```python
from build123d import *

# Parameters (mm, degrees)
SKETCH2_W           = 190
SKETCH2_H           = 22
BOSS_EXTRUDE1_DEPTH = 32
SKETCH3_R           = 0.75
SKETCH3_R_2         = 6
SKETCH3_R_3         = 3
SKETCH3_W           = 25
SKETCH3_H           = 4
CUT_EXTRUDE1_DEPTH  = 24
SKETCH4_W           = 25
SKETCH4_H           = 4
CUT_EXTRUDE2_DEPTH  = 9
SKETCH5_R           = 3
SKETCH5_R_2         = 2
SKETCH5_R_3         = 6.5
CUT_EXTRUDE3_DEPTH  = 24


with BuildPart() as part:
    # Sketch2 → Boss-Extrude1 (new body)
    with BuildSketch(Plane(origin=(0, 0, 0), x_dir=(1, 0, 0), z_dir=(0, 1, 0))):
        Rectangle(SKETCH2_W, SKETCH2_H)
    extrude(amount=BOSS_EXTRUDE1_DEPTH)

    # Sketch3 → Cut-Extrude1 (cut)
    with BuildSketch(Plane(origin=(0, 32, 0), x_dir=(1, 0, 0), z_dir=(0, 1, 0))):
        with Locations((-87, 0)):
            Circle(SKETCH3_R)
        with Locations((-63, 0)):
            Circle(SKETCH3_R_2)
        with Locations((-37, 5)):
            Circle(SKETCH3_R_3)
        with Locations((-43, 0)):
            Circle(SKETCH3_R)
        with Locations((11, 0)):
            Circle(SKETCH3_R_2)
        with Locations((37, 5)):
            Circle(SKETCH3_R_3)
        with Locations((79.5, 9)):
            Rectangle(SKETCH3_W, SKETCH3_H)
    extrude(amount=-CUT_EXTRUDE1_DEPTH, mode=Mode.SUBTRACT)

    # Sketch4 → Cut-Extrude2 (cut, through all)
    with BuildSketch(Plane(origin=(0, 8, 0), x_dir=(1, 0, 0), z_dir=(0, 1, 0))):
        with Locations((79.5, 9)):
            Rectangle(SKETCH4_W, SKETCH4_H)
    extrude(amount=-CUT_EXTRUDE2_DEPTH, mode=Mode.SUBTRACT)

    # Sketch5 → Cut-Extrude3 (cut)
    with BuildSketch(Plane.XY.offset(11)):
        with Locations((-87, 22)):
            Circle(SKETCH5_R)
        with Locations((-63, 20)):
            Circle(SKETCH5_R_2)
        with Locations((11, 20)):
            Circle(SKETCH5_R_2)
        with Locations((79.5, 20)):
            Circle(SKETCH5_R_3)
    extrude(amount=-CUT_EXTRUDE3_DEPTH, mode=Mode.SUBTRACT)


solid = part.part
```
Geometry check sheet. Reference: the model listing, model coordinates, mm. A direction names the side the tool comes from. Round coordinates to 2 decimals unless told otherwise and drop trailing zeros. Loops run counter-clockwise (first coordinate to the right, second up) from the corner with the lowest first, then second, coordinate; pieces in that order, holes last. Notation, with made-up numbers: (61, 57.5) -> (97, 57.5) arc R27 ccw to (97, 78.5) -> close; hole circle Ø7 at (54.25, 76.25). An arc over 180 degrees is marked (long way). Use a Markdown table: item, result.
(1) Sectioned sample at B-B (y = 3.5). Enter the section's corners in (x, z).
Calculated:
| item | result |
|---|---|
| outline | (-95, -11) -> (67, -11) -> (67, -7) -> (92, -7) -> (92, -11) -> (95, -11) -> (95, 11) -> (-95, 11) -> close |
(2) Mould release check, pull along X, two halves, no side actions. Record for faces 4 (the flat face through (95, 16, 0)), 5 (the flat face through (-95, 16, 0)), 6 (the flat face through (-1, 32, 0)), 7 (the cylindrical face through (11, 18, 8)): released by +X, released by -X, zero draft, split by the parting line, or undercut.
Calculated:
| item | result |
|---|---|
| face 4 | released by +X |
| face 5 | released by -X |
| face 6 | zero draft |
| face 7 | undercut |
(3) Set-up check for faces 1 (the flat face through (-37, 8, -5)), 2 (the cylindrical face through (-62.077, 18.226, 8.366)), 3 (the flat face through (92, 16, -9)): record each of +Z, -Z, +X, -X, +Y, -Y from which the full face is reachable in a straight line by a thin tool's end or side.
Calculated:
| item | result |
|---|---|
| face 1 | +Y |
| face 2 | +Z, -Z |
| face 3 | -Z, +Y, -Y |
(4) Sectioned sample at C-C (x = 37). Enter the section's corners in (y, z).
Calculated:
| item | result |
|---|---|
| outline | (0, -11) -> (32, -11) -> (32, -8) -> (8, -8) -> (8, -2) -> (32, -2) -> (32, 11) -> (0, 11) -> close |
(5) Sectioned sample at A-A (x = 11). Enter the section's corners in (y, z), then the cut area to 3 significant figures.
Calculated:
| item | result |
|---|---|
| outline | (0, -11) -> (18, -11) -> (18, -6) -> (8, -6) -> (8, 6) -> (18, 6) -> (18, 11) -> (0, 11) -> close; (22, -11) -> (32, -11) -> (32, -6) -> (22, -6) -> close; (22, 6) -> (32, 6) -> (32, 11) -> (22, 11) -> close |
| area | 376 mm² |
(6) Go/stop test with flat-tipped pins: P1, Ø1.2, axis at x = -43, z = 0, coming from the -Y side; P2, Ø9.5, axis at x = -63.5, z = 1, coming from the +Y side. Record where each tip stops, or that it passes through.
Calculated:
| item | result |
|---|---|
| P1 | y = 0 |
| P2 | y = 8 |
(7) Scan lines: probe 1 along X at (y, z) = (12, 0); probe 2 along X at (y, z) = (16, -5); probe 3 along Z at (x, y) = (37, 25.75). Record each from-to range of solid material in increasing order.
Calculated:
| item | result |
|---|---|
| probe 1 | -95 to -87.75, -86.25 to -69, -57 to -43.75, -42.25 to 5, 17 to 95 |
| probe 2 | -95 to -66.32, -59.68 to -40, -34 to 7.68, 14.32 to 34, 40 to 74.38, 84.62 to 95 |
| probe 3 | -11 to -8, -2 to 11 |
